from build123d import *

# Parameters (mm, degrees)
POCKET_DEPTH = 1.25


with BuildPart() as part:
    # Sketch (on DatumPlane) → Revolution (revolve)
    with BuildSketch(Plane.YZ):
        Polygon((0, 0), (0, -2.5), (19.75, -2.5), (20, -2.25), (20, -0.25), (19.75, 0), align=None)
    revolve(axis=Axis((0, 0, 0), (0, 0, 1)))

    # Sketch005 → Pocket (cut)
    with BuildSketch(Plane.XY):
        with BuildLine():
            add(Edge.make_bspline(
                [(-10.613193, -11.526321), (-12.449243, -11.162413), (-13.862224, -9.91866), (-14.8542, -8.377039)],
                knots=[0, 0, 0, 0, 1, 1, 1, 1], degree=3))
            add(Edge.make_bspline(
                [(-14.8542, -8.377039), (-15.897082, -6.624915), (-15.8448, -4.092006), (-14.308682, -2.612985)],
                knots=[0, 0, 0, 0, 1, 1, 1, 1], degree=3))
            add(Edge.make_bspline(
                [(-14.308682, -2.612985), (-12.954862, -1.221329), (-10.995675, 0.366382), (-8.928485, -0.344235)],
                knots=[0, 0, 0, 0, 1, 1, 1, 1], degree=3))
            add(Edge.make_bspline(
                [(-8.928485, -0.344235), (-7.548524, -1.279114), (-6.005527, -2.671458), (-6.01791, -4.473111)],
                knots=[0, 0, 0, 0, 1, 1, 1, 1], degree=3))
            add(Edge.make_bspline(
                [(-6.01791, -4.473111), (-5.914034, -6.321544), (-7.637953, -7.986302), (-9.425849, -8.055094)],
                knots=[0, 0, 0, 0, 1, 1, 1, 1], degree=3))
            add(Edge.make_bspline(
                [(-9.425849, -8.055094), (-9.389389, -7.319711), (-7.594615, -6.666878), (-8.001174, -5.032388)],
                knots=[0, 0, 0, 0, 1, 1, 1, 1], degree=3))
            add(Edge.make_bspline(
                [(-8.001174, -5.032388), (-8.209612, -2.917044), (-11.141513, -2.729243), (-12.207096, -4.213767)],
                knots=[0, 0, 0, 0, 1, 1, 1, 1], degree=3))
            add(Edge.make_bspline(
                [(-12.207096, -4.213767), (-13.077311, -5.946629), (-12.062634, -8.460277), (-10.019521, -8.718245)],
                knots=[0, 0, 0, 0, 1, 1, 1, 1], degree=3))
            add(Edge.make_bspline(
                [(-10.019521, -8.718245), (-7.773473, -8.716182), (-5.696653, -7.366489), (-4.322883, -5.649449)],
                knots=[0, 0, 0, 0, 1, 1, 1, 1], degree=3))
            add(Edge.make_bspline(
                [(-4.322883, -5.649449), (-3.1947, -4.547406), (-2.959432, -2.923923), (-2.652621, -1.448342)],
                knots=[0, 0, 0, 0, 1, 1, 1, 1], degree=3))
            add(Edge.make_bspline(
                [(-2.652621, -1.448342), (-2.604467, 1.053611), (-4.534073, 2.986657), (-5.257762, 5.279483)],
                knots=[0, 0, 0, 0, 1, 1, 1, 1], degree=3))
            add(Edge.make_bspline(
                [(-5.257762, 5.279483), (-6.18301, 7.323972), (-6.332976, 9.661513), (-5.85281, 11.836705)],
                knots=[0, 0, 0, 0, 1, 1, 1, 1], degree=3))
            add(Edge.make_bspline(
                [(-5.85281, 11.836705), (-5.219238, 14.911693), (-2.105039, 17.205895), (1.027733, 16.779387)],
                knots=[0, 0, 0, 0, 1, 1, 1, 1], degree=3))
            add(Edge.make_bspline(
                [(1.027733, 16.779387), (2.809437, 16.661065), (4.590454, 15.669777), (5.22884, 13.935539)],
                knots=[0, 0, 0, 0, 1, 1, 1, 1], degree=3))
            add(Edge.make_bspline(
                [(5.22884, 13.935539), (6.083921, 12.490226), (6.185045, 10.524848), (5.398756, 9.035509)],
                knots=[0, 0, 0, 0, 1, 1, 1, 1], degree=3))
            add(Edge.make_bspline(
                [(5.398756, 9.035509), (4.309096, 6.612666), (0.749127, 6.126997), (-1.146084, 7.848852)],
                knots=[0, 0, 0, 0, 1, 1, 1, 1], degree=3))
            add(Edge.make_bspline(
                [(-1.146084, 7.848852), (-2.186902, 8.648899), (-2.355441, 11.196255), (-1.629001, 11.847712)],
                knots=[0, 0, 0, 0, 1, 1, 1, 1], degree=3))
            add(Edge.make_bspline(
                [(-1.629001, 11.847712), (-1.774152, 9.981394), (0.165086, 8.70806), (1.874559, 9.327873)],
                knots=[0, 0, 0, 0, 1, 1, 1, 1], degree=3))
            add(Edge.make_bspline(
                [(1.874559, 9.327873), (3.897722, 10.123793), (3.29717, 13.759432), (1.072448, 13.755305)],
                knots=[0, 0, 0, 0, 1, 1, 1, 1], degree=3))
            add(Edge.make_bspline(
                [(1.072448, 13.755305), (0.173341, 13.722285), (-0.871605, 13.870187), (-1.571216, 13.188462)],
                knots=[0, 0, 0, 0, 1, 1, 1, 1], degree=3))
            add(Edge.make_bspline(
                [(-1.571216, 13.188462), (-3.233223, 12.063718), (-3.118341, 9.730992), (-2.769567, 7.980932)],
                knots=[0, 0, 0, 0, 1, 1, 1, 1], degree=3))
            add(Edge.make_bspline(
                [(-2.769567, 7.980932), (-2.618913, 5.918558), (-1.363465, 4.114841), (0.414111, 3.107043)],
                knots=[0, 0, 0, 0, 1, 1, 1, 1], degree=3))
            add(Edge.make_bspline(
                [(0.414111, 3.107043), (2.142158, 1.763541), (4.421226, 2.393673), (6.42444, 2.022886)],
                knots=[0, 0, 0, 0, 1, 1, 1, 1], degree=3))
            add(Edge.make_bspline(
                [(6.42444, 2.022886), (9.702363, 1.669297), (13.188725, 0.387708), (14.958046, -2.571022)],
                knots=[0, 0, 0, 0, 1, 1, 1, 1], degree=3))
            add(Edge.make_bspline(
                [(14.958046, -2.571022), (15.879167, -3.908332), (15.943143, -5.767771), (15.711315, -7.179376)],
                knots=[0, 0, 0, 0, 1, 1, 1, 1], degree=3))
            add(Edge.make_bspline(
                [(15.711315, -7.179376), (15.293062, -8.96108), (13.910349, -10.488943), (12.295809, -11.25941)],
                knots=[0, 0, 0, 0, 1, 1, 1, 1], degree=3))
            add(Edge.make_bspline(
                [(12.295809, -11.25941), (10.784456, -11.658401), (9.026141, -11.801488), (7.59321, -10.84666)],
                knots=[0, 0, 0, 0, 1, 1, 1, 1], degree=3))
            add(Edge.make_bspline(
                [(7.59321, -10.84666), (6.360463, -10.31146), (5.127029, -9.159888), (5.055485, -7.085131)],
                knots=[0, 0, 0, 0, 1, 1, 1, 1], degree=3))
            add(Edge.make_bspline(
                [(5.055485, -7.085131), (4.894513, -5.302051), (6.327443, -3.829909), (7.789954, -3.048436)],
                knots=[0, 0, 0, 0, 1, 1, 1, 1], degree=3))
            add(Edge.make_bspline(
                [(7.789954, -3.048436), (8.789497, -2.372214), (11.444168, -3.280264), (11.127726, -4.213767)],
                knots=[0, 0, 0, 0, 1, 1, 1, 1], degree=3))
            add(Edge.make_bspline(
                [(11.127726, -4.213767), (9.994039, -4.193129), (8.607887, -4.069304), (8.057554, -5.329568)],
                knots=[0, 0, 0, 0, 1, 1, 1, 1], degree=3))
            add(Edge.make_bspline(
                [(8.057554, -5.329568), (6.780093, -7.11196), (8.882366, -9.234871), (10.778952, -8.789789)],
                knots=[0, 0, 0, 0, 1, 1, 1, 1], degree=3))
            add(Edge.make_bspline(
                [(10.778952, -8.789789), (12.699616, -8.657709), (13.124748, -6.510721), (12.787669, -4.964284)],
                knots=[0, 0, 0, 0, 1, 1, 1, 1], degree=3))
            add(Edge.make_bspline(
                [(12.787669, -4.964284), (12.654213, -3.091775), (10.855999, -2.381845), (9.317129, -1.790236)],
                knots=[0, 0, 0, 0, 1, 1, 1, 1], degree=3))
            add(Edge.make_bspline(
                [(9.317129, -1.790236), (7.320795, -1.069988), (5.038288, -0.887002), (3.10249, -1.903743)],
                knots=[0, 0, 0, 0, 1, 1, 1, 1], degree=3))
            add(Edge.make_bspline(
                [(3.10249, -1.903743), (1.208655, -2.416928), (0.529681, -4.319018), (-0.537277, -5.737502)],
                knots=[0, 0, 0, 0, 1, 1, 1, 1], degree=3))
            add(Edge.make_bspline(
                [(-0.537277, -5.737502), (-1.750762, -8.018634), (-3.806945, -9.818224), (-6.083262, -10.982867)],
                knots=[0, 0, 0, 0, 1, 1, 1, 1], degree=3))
            add(Edge.make_bspline(
                [(-6.083262, -10.982867), (-7.501058, -11.543519), (-9.103216, -11.909491), (-10.613193, -11.526321)],
                knots=[0, 0, 0, 0, 1, 1, 1, 1], degree=3))
        make_face()
        with BuildLine():
            add(Edge.make_bspline(
                [(0.564077, -1.502687), (1.337296, -0.694385), (4.170825, 0.71378), (1.582882, 1.072873)],
                knots=[0, 0, 0, 0, 1, 1, 1, 1], degree=3))
            add(Edge.make_bspline(
                [(1.582882, 1.072873), (0.330186, 1.492502), (-2.344434, 3.04169), (-1.386854, 0.466818)],
                knots=[0, 0, 0, 0, 1, 1, 1, 1], degree=3))
            add(Edge.make_bspline(
                [(-1.386854, 0.466818), (-0.974792, -0.71571), (-1.355898, -3.613903), (0.564077, -1.502687)],
                knots=[0, 0, 0, 0, 1, 1, 1, 1], degree=3))
        make_face(mode=Mode.SUBTRACT)
    extrude(amount=-POCKET_DEPTH, mode=Mode.SUBTRACT)


solid = part.part
The model under review builds one solid part; all positions refer to its coordinate system, in mm. Give positions to 0.01 mm unless a question says otherwise; leave off trailing zeros. Order: outer loops, then holes, each group sorted by start corner. A loop starts at its lowest first (then second) coordinate and runs counter-clockwise, first axis right, second up. Notation, with made-up numbers: (-10.5, 81.25) -> (-4.5, 81.25) arc R23 ccw to (-4.5, 109.25) -> close; hole circle Ø4 at (35, -12). An arc over 180 degrees is marked (long way). Write item = value, one per line. Start each with the question number.
(1) Take a section at A-A (z = -1.8). Write out the cut boundary in (x, y), plus the area to 3 significant figures.
(2) For L1, parallel to Y at x = 8, z = -1.05; L2, parallel to X at y = 13.5, z = -1; L3, parallel to X at y = -9.5, z = -0.8, list the stretches that pass through material, from the lowest coordinate up. Write a range as from..to.
(3) Draft analysis for pull direction Y (two halves, no side actions). For faces 1 (the flat face through (2, -1, -1.25)), 2 (the flat face through (0, 0, -2.5)), 3 (the cylindrical face through (19.524, -4.336, -1.236)), state which applies: +Y half, -Y half, draft (parallel to the pull), parting line (faces both ways), or undercut.
(4) For pin 1 Ø1.5 at (y, z) = (11.5, -1.5) entering from +X; pin 2 Ø14.5 at (x, y) = (-1, 1.5) entering from +Z, all flat-tipped, find the tip position at first contact; note any pin that passes through.
Returned:
q1.outline = circle Ø40 at (0, 0)
q1.area = 1,260 mm²
q2.L1 = -18.33..-11.08, -7.59..-5.41, -2.94..-1.41, 1.78..18.33
q2.L2 = -14.76..-5.24, -1.13..2.02, 5.46..14.76
q2.L3 = -17.6..-14, -3.76..5.86, 14.53..17.6
q3.face_1 = undercut
q3.face_2 = draft
q3.face_3 = parting line
q4.pin_1 = 16.87
q4.pin_2 = 0
